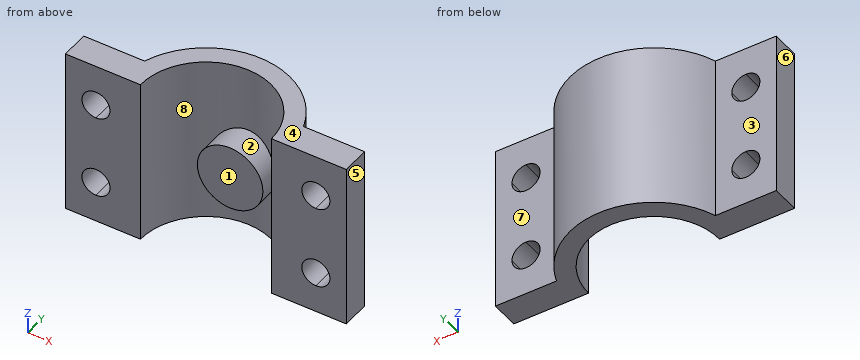
from build123d import *

# Parameters (mm, degrees)
EXTRUDE_1_DEPTH      = 18
EXTRUDE_2_REACH      = 37.341
EXTRUDE_2_END_RADIUS = 7
SKETCH_3_R           = 3.5
CUT_EXTRUDE_1_DEPTH  = 3


with BuildPart() as part:
    # 草图1 → 凸台-拉伸1 (new body)
    with BuildSketch(Plane.XY):
        with BuildLine():
            Line((0, 0), (8, 0))
            ThreePointArc((8, 0), (15, 7), (22, 0))
            Line((22, 0), (30, 0))
            Line((30, 0), (30, 3))
            Line((30, 3), (23.485281374, 3))
            ThreePointArc((23.485281374, 3), (15, 9), (6.514718626, 3))
            Line((6.514718626, 3), (0, 3))
            Line((0, 3), (0, 0))
        make_face()
    extrude(amount=EXTRUDE_1_DEPTH)

    # 凸台-拉伸2: up to this cylinder (the profile starts inside it)
    extrude_2_end = Plane(origin=(15, 0, 7.5), z_dir=(0, 0, -1)) * Cylinder(EXTRUDE_2_END_RADIUS, 89.682, mode=Mode.PRIVATE)
    # 草图3 → 凸台-拉伸2 (add, up to the surface)
    with BuildSketch(Plane(origin=(0, 4, 0), x_dir=(1, 0, 0), z_dir=(0, 1, 0)), mode=Mode.PRIVATE) as extrude_2_sk1:
        with Locations(Location((15, -7.5, 0), (0, 0, 90))):
            Circle(SKETCH_3_R)
    extrude_2_tool1 = extrude(extrude_2_sk1.sketch, amount=EXTRUDE_2_REACH, mode=Mode.PRIVATE) & extrude_2_end
    add(extrude_2_tool1.solids().sort_by_distance((15, 4, 7.5))[0])

    # 草图4 → 切除-拉伸1 (cut)
    with BuildSketch(Plane(origin=(0, 3, 0), x_dir=(1, 0, 0), z_dir=(0, 1, 0))):
        with BuildLine():
            ThreePointArc((4.757359313, -4.5), (4.318019485, -3.439339828), (3.257359313, -3))
            Line((3.257359313, -3), (3.257359313, -6))
            ThreePointArc((3.257359313, -6), (4.318019485, -5.560660172), (4.757359313, -4.5))
        make_face()
        with BuildLine():
            Line((3.257359313, -6), (3.257359313, -3))
            ThreePointArc((3.257359313, -3), (1.757359313, -4.5), (3.257359313, -6))
        make_face()
        with BuildLine():
            ThreePointArc((4.757359313, -13.5), (4.318019485, -12.439339828), (3.257359313, -12))
            Line((3.257359313, -12), (3.257359313, -15))
            ThreePointArc((3.257359313, -15), (4.318019485, -14.560660172), (4.757359313, -13.5))
        make_face()
        with BuildLine():
            Line((3.257359313, -15), (3.257359313, -12))
            ThreePointArc((3.257359313, -12), (1.757359313, -13.5), (3.257359313, -15))
        make_face()
        with BuildLine():
            ThreePointArc((28.242640687, -4.5), (27.803300859, -3.439339828), (26.742640687, -3))
            Line((26.742640687, -3), (26.742640687, -6))
            ThreePointArc((26.742640687, -6), (27.803300859, -5.560660172), (28.242640687, -4.5))
        make_face()
        with BuildLine():
            Line((26.742640687, -6), (26.742640687, -3))
            ThreePointArc((26.742640687, -3), (25.242640687, -4.5), (26.742640687, -6))
        make_face()
        with BuildLine():
            ThreePointArc((28.242640687, -13.5), (27.803300859, -12.439339828), (26.742640687, -12))
            Line((26.742640687, -12), (26.742640687, -15))
            ThreePointArc((26.742640687, -15), (27.803300859, -14.560660172), (28.242640687, -13.5))
        make_face()
        with BuildLine():
            Line((26.742640687, -15), (26.742640687, -12))
            ThreePointArc((26.742640687, -12), (25.242640687, -13.5), (26.742640687, -15))
        make_face()
    extrude(amount=-CUT_EXTRUDE_1_DEPTH, mode=Mode.SUBTRACT)


solid = part.part
Source: CAD feature listing. Evaluate the final solid. Frame: model axes, mm. Face numbers are marked on the shaded views. A direction names the side the tool comes from. Round coordinates to 2 decimals unless told otherwise and drop trailing zeros. Loops run counter-clockwise (first coordinate to the right, second up) from the corner with the lowest first, then second, coordinate; pieces in that order, holes last. Notation, with made-up numbers: (10, 38) -> (63, 38) arc R16 cw to (63, 62) -> close; hole circle Ø4 at (-27.75, 28). An arc over 180 degrees is marked (long way). Answer as a JSON object with one key per item and string values. Group by question number.
Q1. Mould query, pull axis X, two halves, no side actions, for the marked faces 6, 7 and 8. Classes: pulls with the +X half, pulls with the -X half, needs draft (parallel to the pull), parting line crosses it, or undercut.
Q2. Ray query, line 1 (X direction, y = 2.75, z = 13); line 2 (X direction, y = 6.25, z = 10); line 3 (Y direction, x = 15, z = 15.75). Return the intervals inside material, ascending. Write a range as from..to.
Q3. Section query A-A (y = 1.75). Output: boundary loops of the cut face in (x, z).
Q4. Section query C-C (z = 14). Output: boundary loops of the cut face in (x, y), plus the area to 3 significant figures.
Q5. Access query for the marked faces 1, 2, 3, 4 and 5. Directions: +Z, -Z, +X, -X, +Y, -Y. A direction counts if a zero-diameter tool reaches every point of the face in a straight line with its end or side. Return the directions, or none.
Q6. Section query B-B (y = 5.5). Output: boundary loops of the cut face in (x, z), plus the area to 3 significant figures.
Q7. Contact query for flat-ended pins moving along their axis: P1, Ø2, axis at x = 27, z = 11.5, coming from the +Y side; P2, Ø5.5, axis at x = 14, z = 6.5, coming from the -Y side; P3, Ø1, axis at x = 14.5, y = 2.5, coming from the -Z side; P4, Ø5, axis at y = 8, z = 11, coming from the -X side. Output: stop coordinate, or through.
Q8. Section query D-D (x = 15). Output: boundary loops of the cut face in (y, z).
Completed:
{
 "1": {"face 6": "pulls with the -X half", "face 7": "needs draft", "face 8": "undercut"},
 "2": {"line 1": "0..1.84, 4.67..8.56, 21.44..25.33, 28.16..30", "line 2": "8.52..11.85, 12.55..17.45, 18.15..21.48", "line 3": "7..9"},
 "3": {"outline": "(0, 0) -> (8.22, 0) -> (8.22, 18) -> (0, 18) -> close; (21.78, 0) -> (30, 0) -> (30, 18) -> (21.78, 18) -> close; hole circle Ø3 at (3.26, 4.5); hole circle Ø3 at (3.26, 13.5); hole circle Ø3 at (26.74, 4.5); hole circle Ø3 at (26.74, 13.5)"},
 "4": {"outline": "(0, 0) -> (1.84, 0) -> (1.84, 3) -> (0, 3) -> close; (4.67, 0) -> (8, 0) arc R7 cw to (22, 0) -> (25.33, 0) -> (25.33, 3) -> (23.49, 3) arc R9 ccw to (6.51, 3) -> (4.67, 3) -> close; (28.16, 0) -> (30, 0) -> (30, 3) -> (28.16, 3) -> close", "area": "70.3 mm²"},
 "5": {"face 1": "+Z, -Z, -Y", "face 2": "-Y", "face 3": "+Z, -Z, -X, +Y", "face 4": "+Z, +X, -X, +Y, -Y", "face 5": "+Z, -Z, +X, +Y, -Y"},
 "6": {"outline": "(7.88, 0) -> (10.67, 0) -> (10.67, 18) -> (7.88, 18) -> close; circle Ø7 at (15, 7.5); (19.33, 0) -> (22.12, 0) -> (22.12, 18) -> (19.33, 18) -> close", "area": "139 mm²"},
 "7": {"P1": "y = 3", "P2": "y = 4", "P3": "through", "P4": "x = 7.88"},
 "8": {"outline": "(4, 4) -> (7, 4) -> (7, 0) -> (9, 0) -> (9, 18) -> (7, 18) -> (7, 11) -> (4, 11) -> close"}
}
